```python
from build123d import *

# Parameters (mm, degrees)
F0_W       = 152.4
F0_H       = 279.4
F0_R       = 9.525
F1_DEPTH   = 25.4
F2_SIZE2   = 50.8
F2_SIZE    = 127
F2_2_SIZE2 = 50.8
F2_2_SIZE  = 127


with BuildPart() as f1:
    # F0 (on Front) → F1 (new body)
    with BuildSketch(Plane.XZ):
        with Locations((0.297114253, 69.4026991844)):
            Rectangle(F0_W, F0_H)
        with Locations((0, 167.8276991844)):
            Circle(F0_R, mode=Mode.SUBTRACT)
    extrude(amount=F1_DEPTH)

    # F2
    f2_edges = [f1.edges().sort_by_distance(p)[0] for p in [
        (-75.902886, -12.7, 209.102699),
    ]]
    f2_side = f1.faces().sort_by_distance((-75.902886, -12.7, 69.402699))[0]
    chamfer(f2_edges, length=F2_SIZE, length2=F2_SIZE2, reference=f2_side)

    # F2#2
    f2_2_edges = [f1.edges().sort_by_distance(p)[0] for p in [
        (76.497114, -12.7, 209.102699),
    ]]
    f2_2_side = f1.faces().sort_by_distance((76.497114, -12.7, 69.402699))[0]
    chamfer(f2_2_edges, length=F2_2_SIZE, length2=F2_2_SIZE2, reference=f2_2_side)


solid = f1.part
```
Model file for the job. Use its own axes, mm. Coordinates: 2 decimals unless noted, no trailing zeros. Write each loop counter-clockwise with the first axis right and the second up, starting at its lowest first coordinate (ties: lowest second). Pieces come first, ordered by that corner, then holes. Notation, with made-up numbers: (36, -33) - (71, -33) arc R11 ccw to (71, -14) - close; hole circle Ø11 at (74.25, -11.75). An arc over 180 degrees is marked (long way). One line per question, with ' | ' between items. Start each with the question number.
Q1. Pin check, flat tip, straight feed: pin 1 (4 mm diameter, centred on x = 37, y = -14, fed in from +Z). Stop position of the tip, or through.
Q2. Pull direction Z, two halves, no side cores. Call faces 1 (the face through (-1, 0, 40)), 2 (the face through (-2.06, -12.52, 158.53)), 3 (the face through (0, -13, 209.103)): pulls with the +Z half, pulls with the -Z half, needs draft (parallel to the pull), parting line crosses it, or undercut.
Q3. Cut at C-C, the plane x = -47.5. List the corners of the cut face in (y, z).
Q4. Cut at B-B, the plane y = -22.75. List the corners of the cut face in (x, z) (3 decimals).
Q5. Drill centre lines: line 1 (Z direction, x = 0, y = -13.25); line 2 (X direction, y = -18.75, z = 166); line 3 (Z direction, x = -7, y = -17.25). Where is each one in solid material? Low to high. Write a range as [from, to].
Q6. Cut at A-A, the plane x = 0. List the corners of the cut face in (y, z), then the cut area to 3 significant figures.
Q7. Cut at D-D, the plane x = -63. List the corners of the cut face in (y, z).
Answer below:
1) pin 1: z = 185.85
2) face 1: needs draft | face 2: undercut | face 3: pulls with the +Z half
3) outline: (-25.4, -70.3) - (0, -70.3) - (0, 153.11) - (-25.4, 153.11) - close
4) outline: (-75.903, -70.297) - (76.497, -70.297) - (76.497, 82.103) - (25.697, 209.103) - (-25.103, 209.103) - (-75.903, 82.103) - close; hole circle Ø19.05 at (0, 167.828)
5) line 1: [-70.3, 158.3], [177.35, 209.1] | line 2: [-42.34, -9.35], [9.35, 42.94] | line 3: [-70.3, 161.37], [174.29, 209.1]
6) outline: (-25.4, -70.3) - (0, -70.3) - (0, 158.3) - (-25.4, 158.3) - close; (-25.4, 177.35) - (0, 177.35) - (0, 209.1) - (-25.4, 209.1) - close | area: 6,610 mm^2
7) outline: (-25.4, -70.3) - (0, -70.3) - (0, 114.36) - (-25.4, 114.36) - close
